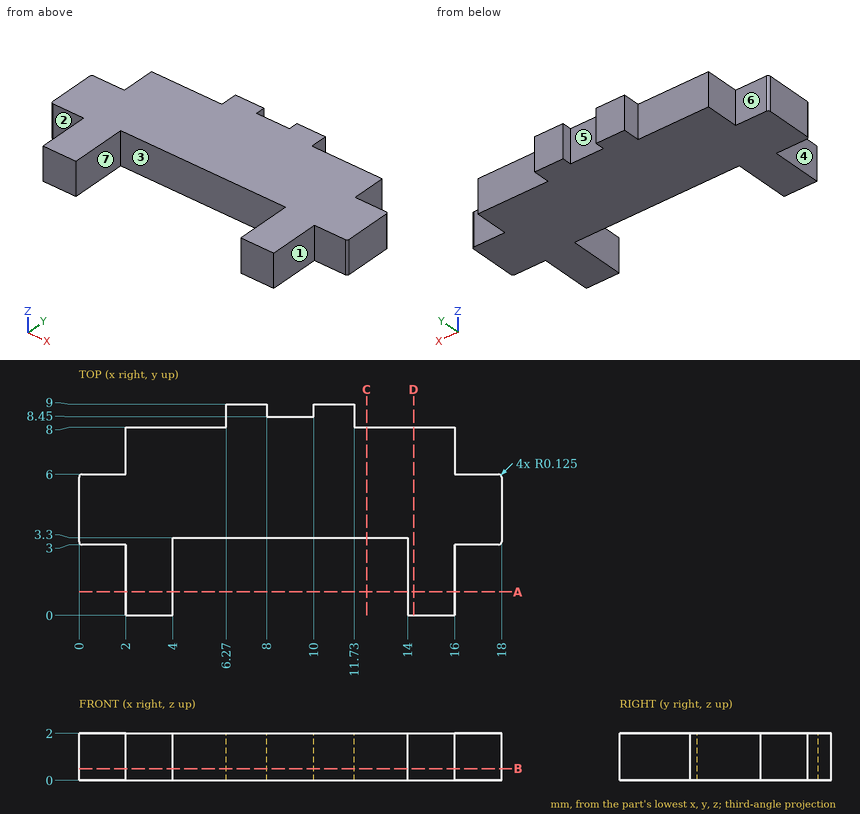
Can you work these out from the drawing? Everything is in mm from the part's minimum corner. A direction names the side the tool comes from. Give positions to 0.01 mm unless a question says otherwise; leave off trailing zeros. Order: outer loops, then holes, each group sorted by start corner. A loop starts at its lowest first (then second) coordinate and runs counter-clockwise, first axis right, second up. Notation, with made-up numbers: M 81,80.25 L 125,80.25 A12 cw 125,95.25 Z; hole C 13.25,62 d11. An arc over 180 degrees is marked long. Use a Markdown table: item, result. Add a question column.
Item 1: Suppose I cut it at B-B (z = 0.5). List the corners of the cut face in (x, y) for me (3 decimals).
Item 2: If I drill on L1, parallel to X at y = 2.25, z = 1.95; L2, parallel to X at y = 7, z = 1.8; L3, parallel to X at y = 8.75, z = 0.85, over which ranges is the centre line in solid material (lowest first)? Write a range as [from, to].
Item 3: Will these pins go through, and if not, where does the flat tip stop? pin 1 (1 mm diameter, centred on y = 4, z = 0.5, fed in from -X); pin 2 (1.1 mm diameter, centred on y = 8.5, z = 1, fed in from +X); pin 3 (0.9 mm diameter, centred on x = 1, z = 1, fed in from -Y); pin 4 (0.9 mm diameter, centred on x = 17, z = 1, fed in from +Y).
Item 4: We'd pull the mould along X, two halves only. Please class the marked faces 1, 2, 3 and 4: +X half, -X half, draft (parallel to the pull), parting line (faces both ways), or undercut.
Item 5: For the marked faces 5, 6 and 7, which set-ups out of +Z, -Z, +X, -X, +Y, -Y let a thin tool reach every point of the face, with its end or its side?
Item 6: Suppose I cut it at C-C (x = 12.25). List the corners of the cut face in (y, z) for me, then the cut area to 3 significant figures.
Item 7: Suppose I cut it at D-D (x = 14.25). List the corners of the cut face in (y, z) for me, then the cut area to 3 significant figures.
Item 8: Suppose I cut it at A-A (y = 1). List the corners of the cut face in (x, z) for me, then the cut area to 3 significant figures.
Answer sheet:
| question | item | result |
|---|---|---|
| 1 | outline | M 0,3.125 A0.125 ccw 0.125,3 L 2,3 L 2,0 L 4,0 L 4,3.3 L 14,3.3 L 14,0 L 16,0 L 16,3 L 17.875,3 A0.125 ccw 18,3.125 L 18,5.875 A0.125 ccw 17.875,6 L 16,6 L 16,8 L 11.73,8 L 11.73,9 L 10,9 L 10,8.45 L 8,8.45 L 8,9 L 6.27,9 L 6.27,8 L 2,8 L 2,6 L 0.125,6 A0.125 ccw 0,5.875 Z |
| 2 | L1 | x = [2, 4], [14, 16] |
| 2 | L2 | x = [2, 16] |
| 2 | L3 | x = [6.27, 8], [10, 11.73] |
| 3 | pin 1 | stops at x = 0 |
| 3 | pin 2 | stops at x = 16 |
| 3 | pin 3 | stops at y = 3 |
| 3 | pin 4 | stops at y = 6 |
| 4 | face 1 | +X half |
| 4 | face 2 | draft |
| 4 | face 3 | undercut |
| 4 | face 4 | -X half |
| 5 | face 5 | +Z, -Z, +Y |
| 5 | face 6 | +Z, -Z, -X, +Y |
| 5 | face 7 | +Z, -Z, -Y |
| 6 | outline | M 3.3,0 L 8,0 L 8,2 L 3.3,2 Z |
| 6 | area | 9.40 mm² |
| 7 | outline | M 0,0 L 8,0 L 8,2 L 0,2 Z |
| 7 | area | 16.0 mm² |
| 8 | outline | M 2,0 L 4,0 L 4,2 L 2,2 Z; M 14,0 L 16,0 L 16,2 L 14,2 Z |
| 8 | area | 8.00 mm² |
